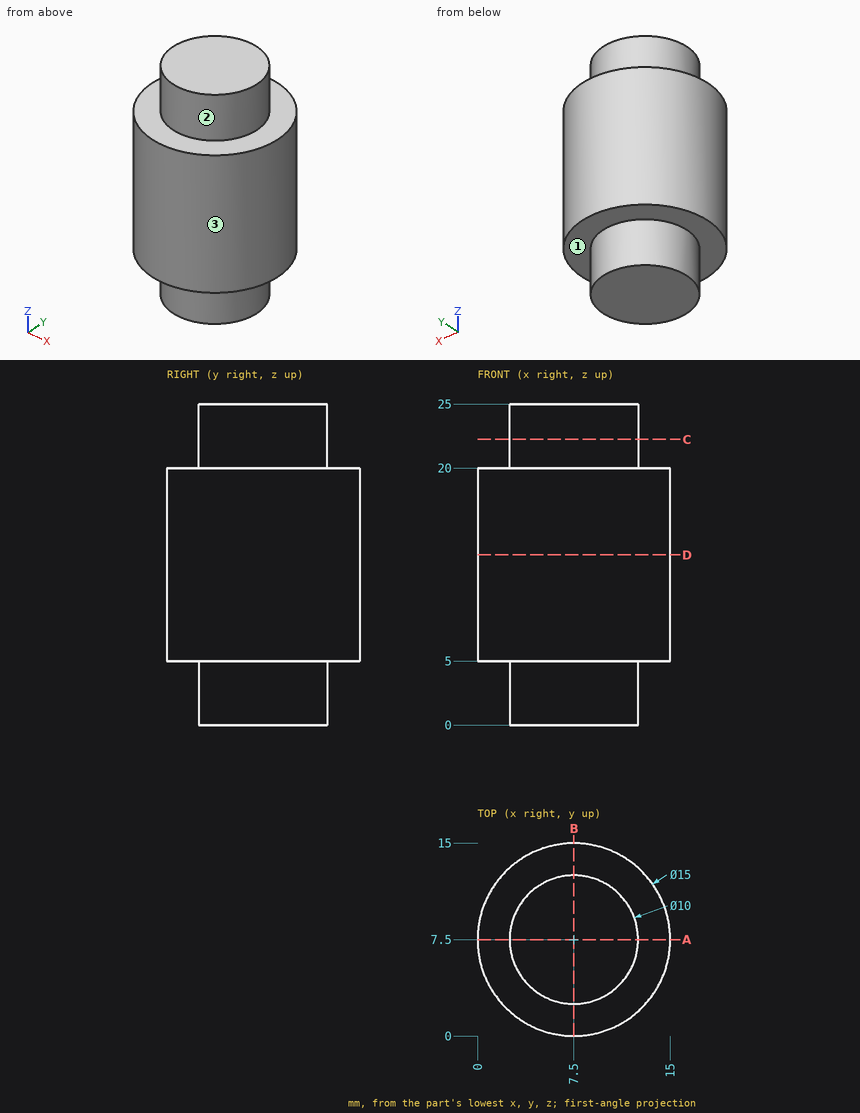
Verification items for this drawing (mm, ordinates from the low corner). A direction names the side the tool comes from. Coordinates: 2 decimals unless noted, no trailing zeros. Order: outer loops, then holes, each group sorted by start corner. A loop starts at its lowest first (then second) coordinate and runs counter-clockwise, first axis right, second up.
Q1. Sectioned sample at C-C on z = 22.25. Record the cut outline in (x, y), and give its area (3 significant figures).
Reply:
outline: circle Ø10 at (7.5, 7.5)
area: 78.5 mm2
Q2. Depth check by flat-ended pin: pin 1 Ø8 at (y, z) = (9.5, 12.5) entering from -X; pin 2 Ø1 at (y, z) = (2.5, 22) entering from +X; pin 3 Ø6 at (y, z) = (11.5, 6.5) entering from -X; pin 4 Ø1 at (y, z) = (2.5, 11) entering from -X. Enter the tip coordinate at first touch or a pass-through.
Reply:
pin 1: stops at x = 0
pin 2: stops at x = 9.68
pin 3: stops at x = 0.07
pin 4: stops at x = 1.5
Q3. Thickness scan on probe 1 along Z at (x, y) = (4, 2.25); probe 2 along X at (y, z) = (10.5, 11.5); probe 3 along X at (y, z) = (7, 15). Record the ranges inside material, lowest first.
Reply:
probe 1: z = 5 to 20
probe 2: x = 0.63 to 14.37
probe 3: x = 0.02 to 14.98
Q4. Tool access check on the marked faces 1, 2 and 3. Record the directions out of +Z, -Z, +X, -X, +Y, -Y that give a thin tool (end or side, any length) a straight path to the whole face; none if there is none.
Reply:
face 1: -Z
face 2: +Z
face 3: +Z, -Z
Q5. Sectioned sample at D-D on z = 13.25. Record the cut outline in (x, y), and give its area (3 significant figures).
Reply:
outline: circle Ø15 at (7.5, 7.5)
area: 177 mm2
Q6. Sectioned sample at A-A on y = 7.5. Record the cut outline in (x, z), and give its area (3 significant figures).
Reply:
outline: (0, 5) - (2.5, 5) - (2.5, 0) - (12.5, 0) - (12.5, 5) - (15, 5) - (15, 20) - (12.5, 20) - (12.5, 25) - (2.5, 25) - (2.5, 20) - (0, 20) - close
area: 325 mm2
